The model under review builds one solid part; all positions refer to its coordinate system, in mm. A direction names the side the tool comes from. Round coordinates to 2 decimals unless told otherwise and drop trailing zeros. Loops run counter-clockwise (first coordinate to the right, second up) from the corner with the lowest first, then second, coordinate; pieces in that order, holes last. Notation, with made-up numbers: M 35.5,71 L 47.5,71 A27 cw 47.5,110 Z; hole C -34,50.25 d3. An arc over 180 degrees is marked long. Answer as a JSON object with one key per item and string values. Group by question number.
Item 1: Tool access review of faces 1 (the face through (240, -340, -10)), 2 (the face through (246.99, -172.69, -97.15)): name each direction out of +Z, -Z, +X, -X, +Y, -Y from which nothing blocks a thin tool from reaching the whole face with its end or side.
Item 2: Consider section C-C (x = 186.5). Give the boundary of the cut face in (y, z).
Item 3: The part is to be moulded in two halves that separate along X. For faces 3 (the face through (250, -177, -44)), 4 (the face through (123, 0, -44)), 5 (the face through (2.85, -346.99, -45.63)), 6 (the face through (123, -173, -90)), say which applies: +X half, -X half, draft (parallel to the pull), parting line (faces both ways), or undercut.
Item 4: Insertion check: P1, Ø8, axis at x = 10, y = -10, coming from the +Z side; P2, Ø6, axis at x = 214.5, y = -227, coming from the +Z side. Each pin has a flat end and moves straight along its axis. Give the tip position at first contact, or say it passes through.
Item 5: To check wall thickness, follow line 1 (Y direction, x = 76, z = -14); line 2 (X direction, y = -64, z = -24.5); line 3 (Z direction, x = 14.5, y = -28.5). State the ranges of each line that lie inside material, in increasing order.
Item 6: Consider section B-B (y = -192). Give the boundary of the cut face in (x, z), and give its area (3 significant figures).
```python
from build123d import *

# Parameters (mm, degrees)
SKETCH1_W           = 250
SKETCH1_H           = 350
BOSS_EXTRUDE1_DEPTH = 100
SKETCH2_W           = 230
SKETCH2_H           = 330
CUT_EXTRUDE1_DEPTH  = 90
FILLET1_R           = 10
SKETCH3_W           = 10
SKETCH3_H           = 10
BOSS_EXTRUDE2_DEPTH = 90
SKETCH4_W           = 10
SKETCH4_H           = 9.995398269
BOSS_EXTRUDE3_DEPTH = 90
SKETCH5_W           = 10
SKETCH5_H           = 10
BOSS_EXTRUDE4_DEPTH = 90
FILLET2_R           = 10
FILLET3_R           = 10
SKETCH6_R           = 4.668020142
CUT_EXTRUDE2_DEPTH  = 10
SKETCH7_R           = 5
CUT_EXTRUDE3_DEPTH  = 10
SKETCH8_R           = 5
CUT_EXTRUDE4_DEPTH  = 10
SKETCH9_R           = 5
CUT_EXTRUDE5_DEPTH  = 10


# Some blends are built 0.0001 mm under size
with BuildPart() as part:
    # Sketch1 → Boss-Extrude1 (new body)
    with BuildSketch(Plane.XY):
        with Locations((125, -175)):
            Rectangle(SKETCH1_W, SKETCH1_H)
    extrude(amount=-BOSS_EXTRUDE1_DEPTH)

    # Sketch2 → Cut-Extrude1 (cut)
    with BuildSketch(Plane.XY):
        with Locations((125, -175)):
            Rectangle(SKETCH2_W, SKETCH2_H)
    extrude(amount=-CUT_EXTRUDE1_DEPTH, mode=Mode.SUBTRACT)

    # Fillet1
    fillet1_edges = [part.edges().sort_by_distance(p)[0] for p in [
        (250, -175, -100),
        (125, 0, -100),
        (0, -175, -100),
        (125, -350, -100),
        (0, 0, -50),
        (250, 0, -50),
        (250, -350, -50),
        (0, -350, -50),
    ]]
    fillet(fillet1_edges, radius=FILLET1_R)

    # Sketch3 → Boss-Extrude2 (add)
    with BuildSketch(Plane.XY.offset(-90)):
        with Locations((15, -335)):
            Rectangle(SKETCH3_W, SKETCH3_H)
    extrude(amount=BOSS_EXTRUDE2_DEPTH)

    # Sketch4 → Boss-Extrude3 (add)
    with BuildSketch(Plane.XY.offset(-90)):
        with Locations((235, -335.002300866)):
            Rectangle(SKETCH4_W, SKETCH4_H)
    extrude(amount=BOSS_EXTRUDE3_DEPTH)

    # Sketch5 → Boss-Extrude4 (add)
    with BuildSketch(Plane.XY.offset(-90)):
        with Locations((235, -15)):
            Rectangle(SKETCH5_W, SKETCH5_H)
        with Locations((15, -15)):
            Rectangle(SKETCH5_W, SKETCH5_H)
    extrude(amount=BOSS_EXTRUDE4_DEPTH)

    # Fillet2
    fillet2_edges = [part.edges().sort_by_distance(p)[0] for p in [
        (230, -20, -45),
    ]]
    fillet(fillet2_edges, radius=FILLET2_R - 0.0001)  # a hair under: the kernel refuses the full size

    # Fillet3
    # the kernel refuses this fillet: 10 mm, written as the material it takes off along each edge
    with BuildSketch(Plane(origin=(230, -330.004601731, -90), x_dir=(1, 0, 0), z_dir=(0, 0, 1))) as fillet3_piece_1:
        with BuildLine():
            CenterArc((9.999998941, -10), FILLET3_R, 90, 89.973634023)
            Line((0, -9.995398269), (0, 0))
            Line((0, 0), (9.999998941, 0))
        make_face()
    extrude(amount=114.999997353, mode=Mode.SUBTRACT)
    with BuildSketch(Plane(origin=(20, -330, -90), x_dir=(0, -1, 0), z_dir=(0, 0, 1))) as fillet3_piece_2:
        with BuildLine():
            CenterArc((FILLET3_R, -FILLET3_R), FILLET3_R, 90, 90)
            Line((0, -FILLET3_R), (0, 0))
            Line((0, 0), (FILLET3_R, 0))
        make_face()
    extrude(amount=115, mode=Mode.SUBTRACT)
    with BuildSketch(Plane(origin=(20, -20, -90), x_dir=(0, 1, 0), z_dir=(0, 0, 1))) as fillet3_piece_3:
        with BuildLine():
            CenterArc((FILLET3_R, FILLET3_R), FILLET3_R, 180, 90)
            Line((0, FILLET3_R), (0, 0))
            Line((0, 0), (FILLET3_R, 0))
        make_face()
    extrude(amount=115, mode=Mode.SUBTRACT)

    # Sketch6 → Cut-Extrude2 (cut)
    with BuildSketch(Plane.XY):
        with Locations((240, -10)):
            Circle(SKETCH6_R)
    extrude(amount=-CUT_EXTRUDE2_DEPTH, mode=Mode.SUBTRACT)

    # Sketch7 → Cut-Extrude3 (cut)
    with BuildSketch(Plane.XY):
        with Locations((10, -10)):
            Circle(SKETCH7_R)
    extrude(amount=-CUT_EXTRUDE3_DEPTH, mode=Mode.SUBTRACT)

    # Sketch8 → Cut-Extrude4 (cut)
    with BuildSketch(Plane.XY):
        with Locations((239.999998941, -340.004601731)):
            Circle(SKETCH8_R)
    extrude(amount=-CUT_EXTRUDE4_DEPTH, mode=Mode.SUBTRACT)

    # Sketch9 → Cut-Extrude5 (cut)
    with BuildSketch(Plane.XY):
        with Locations((10, -340)):
            Circle(SKETCH9_R)
    extrude(amount=-CUT_EXTRUDE5_DEPTH, mode=Mode.SUBTRACT)


solid = part.part
```
Geometry results:
{
 "1": {"face 1": "+Z", "face 2": "-Z, +X, +Y, -Y"},
 "2": {"outline": "M -350,-90 A10 ccw -340,-100 L -10,-100 A10 ccw 0,-90 L 0,0 L -10,0 L -10,-90 L -340,-90 L -340,0 L -350,0 Z"},
 "3": {"face 3": "+X half", "face 4": "draft", "face 5": "-X half", "face 6": "undercut"},
 "4": {"P1": "stops at z = -10", "P2": "stops at z = -90"},
 "5": {"line 1": "y = -350 to -340, -10 to 0", "line 2": "x = 0 to 10, 240 to 250", "line 3": "z = -100 to -90"},
 "6": {"outline": "M 0,-90 A10 ccw 10,-100 L 240,-100 A10 ccw 250,-90 L 250,0 L 240,0 L 240,-90 L 10,-90 L 10,0 L 0,0 Z", "area": "4,260 mm^2"}
}
